```python
from build123d import *

# Parameters (mm, degrees)
SKETCH1_W           = 1.2
SKETCH1_H           = 10
SKETCH1_W_2         = 19
SKETCH1_H_2         = 1.2
BOSS_EXTRUDE1_DEPTH = 389
SKETCH3_R           = 4.05
CUT_EXTRUDE2_DEPTH  = 370
CUT_EXTRUDE4_DEPTH  = 370


with BuildPart() as part:
    # Sketch1 → Boss-Extrude1 (new body)
    with BuildSketch(Plane.XY):
        Rectangle(SKETCH1_W, SKETCH1_H)
        with Locations((0, -5.6)):
            Rectangle(SKETCH1_W_2, SKETCH1_H_2)
        with Locations((0, 5.6)):
            Rectangle(SKETCH1_W_2, SKETCH1_H_2)
    extrude(amount=BOSS_EXTRUDE1_DEPTH)

    # Sketch3 → Cut-Extrude2 (cut)
    with BuildSketch(Plane(origin=(0, 6.2, 0), x_dir=(1, 0, 0), z_dir=(0, 1, 0))):
        with BuildLine():
            Line((-9.5, 0), (-9.5, -9.5))
            ThreePointArc((-9.5, -9.5), (-6.717514436, -2.782485594), (-4.2e-08, 0))
            Line((-4.2e-08, 0), (-9.5, 0))
        make_face()
        with BuildLine():
            Line((9.5, 0), (-4.2e-08, 0))
            ThreePointArc((-4.2e-08, 0), (6.717514406, -2.782485564), (9.5, -9.5))
            Line((9.5, -9.5), (9.5, 0))
        make_face()
        with BuildLine():
            ThreePointArc((14.5, -9.5), (0, 5), (-14.5, -9.5))
            Line((-14.5, -9.5), (-9.5, -9.5))
            Line((-9.5, -9.5), (-9.5, 0))
            Line((-9.5, 0), (-4.2e-08, 0))
            Line((-4.2e-08, 0), (9.5, 0))
            Line((9.5, 0), (9.5, -9.5))
            Line((9.5, -9.5), (14.5, -9.5))
        make_face()
        with Locations((0, -9.5)):
            Circle(SKETCH3_R)
    cut_extrude2 = extrude(amount=-CUT_EXTRUDE2_DEPTH, mode=Mode.SUBTRACT)

    # Mirror1: Cut-Extrude2 across plane
    add(cut_extrude2.mirror(Plane.XY.offset(194.5)), mode=Mode.SUBTRACT)

    # Sketch6 → Cut-Extrude4 (cut)
    with BuildSketch(Plane.ZY.offset(0.6)):
        with BuildLine():
            Line((20, -5), (-1, -5))
            Line((-1, -5), (-1, 5))
            Line((-1, 5), (20, 5))
            Line((20, 5), (20, 4.517635543))
            ThreePointArc((20, 4.517635543), (20.154857723, 3.983094121), (20.571469063, 3.614108434))
            ThreePointArc((20.571469063, 3.614108434), (22.857345314, 0), (20.571469063, -3.614108434))
            ThreePointArc((20.571469063, -3.614108434), (20.154857723, -3.983094121), (20, -4.517635543))
            Line((20, -4.517635543), (20, -5))
        make_face()
    cut_extrude4 = extrude(amount=-CUT_EXTRUDE4_DEPTH, mode=Mode.SUBTRACT)

    # Mirror2: Cut-Extrude4 across plane
    add(cut_extrude4.mirror(Plane.XY.offset(194.5)), mode=Mode.SUBTRACT)


solid = part.part
```
Here's how the part is built. I have some questions about the finished solid (model axes, mm). A direction names the side the tool comes from. Give positions to 0.01 mm unless a question says otherwise; leave off trailing zeros. Write each loop counter-clockwise with the first axis right and the second up, starting at its lowest first coordinate (ties: lowest second). Pieces come first, ordered by that corner, then holes. Notation, with made-up numbers: (-15, -14.75) -> (23, -14.75) arc R33 ccw to (23, 14.25) -> close; hole circle Ø1 at (-39, -16). An arc over 180 degrees is marked (long way). Write each question's results on one line, items separated by ' | '.
Item 1: On a 3-axis mill with a long thin cutter (end or side, diameter ignored), from which of +Z, -Z, +X, -X, +Y, -Y can I reach the whole of each face in a straight line? I mean faces 4 (the face through (0.6, 0, 192)), 5 (the face through (-0.878, -5.592, 375.546)). Say none if no direction works.
Output:
face 4: +Z, -Z, +X | face 5: +Y, -Y
Item 2: Suppose I cut it at B-B on y = -1.5. Write out the boundary of the cut face in (x, z), plus the area to 3 significant figures.
Output:
outline: (-0.6, 22.57) -> (0.6, 22.57) -> (0.6, 366.43) -> (-0.6, 366.43) -> close | area: 413 mm^2
Item 3: If I drill on L1, parallel to Z at x = 0, y = -5.45; L2, parallel to Y at x = 8.25, z = 193.5; L3, parallel to X at y = 5.65, z = 379.5, over which ranges is the centre line in solid material (lowest first)?
Output:
L1: z = 0 to 5.45, 13.55 to 375.45, 383.55 to 389 | L2: y = -6.2 to -5, 5 to 6.2 | L3: x = -9.5 to -4.05, 4.05 to 9.5
Item 4: We'd pull the mould along X, two halves only. Please class faces 1 (the face through (-0.878, 5.608, 375.546)), 2 (the face through (0, -6.2, 192)), 3 (the face through (-0.6, 0, 192)): pulls with the +X half, pulls with the -X half, needs draft (parallel to the pull), parting line crosses it, or undercut.
Output:
face 1: undercut | face 2: needs draft | face 3: pulls with the -X half
Item 5: For pin 1 Ø4 at (x, y) = (6.5, 3.5) entering from -Z; pin 2 Ø5 at (y, z) = (0, 151) entering from +X; pin 3 Ø2 at (y, z) = (-3.5, 94) entering from -X, each with a flat end and sliding along its axis, tell me the tip position at first contact or that it passes through.
Output:
pin 1: stops at z = 1.53 | pin 2: stops at x = 0.6 | pin 3: stops at x = -0.6
Item 6: Suppose I cut it at A-A on z = 326. Write out the boundary of the cut face in (x, y).
Output:
outline: (-9.5, -6.2) -> (9.5, -6.2) -> (9.5, -5) -> (0.6, -5) -> (0.6, 5) -> (9.5, 5) -> (9.5, 6.2) -> (-9.5, 6.2) -> (-9.5, 5) -> (-0.6, 5) -> (-0.6, -5) -> (-9.5, -5) -> close
